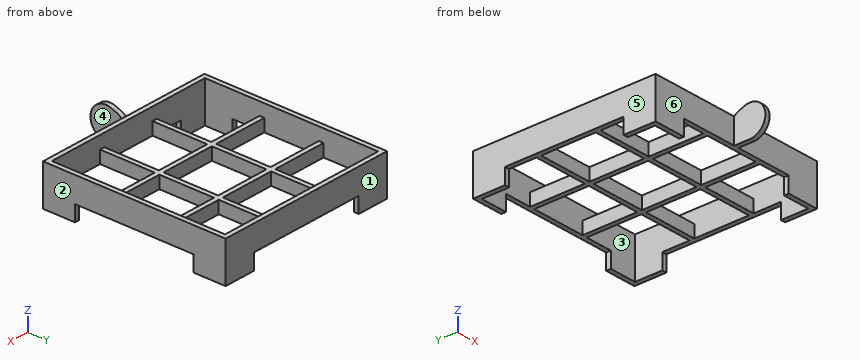
```python
from build123d import *

# Parameters (mm, degrees)
F0_W        = 58.5
F0_H        = 58.5
F0_W_2      = 17.5
F0_H_2      = 17.5
F1_DEPTH    = 4
F2_W        = 1.5
F2_H        = 10
F3_DEPTH    = 10
F4_R        = 4.99999
F6_DEPTH    = 1.5
F7_T1_DEPTH = 26.0435355486
F8_R        = 5
F9_W        = 58.5
F9_H        = 58.5
F9_W_2      = 55.5
F9_H_2      = 55.5
F10_DEPTH   = 4
F12_DEPTH   = 5


# Not quite as in the source:
# - a fillet or chamfer that OpenCascade refuses, or shapes differently, is made with other operations: its cross-section is extruded or revolved along the edge and cut away or added
# - a fillet or chamfer is up to 0.001 mm smaller than in the source, because OpenCascade refuses the exact size


with BuildPart() as f1:
    # F0 (on Top) → F1 (new body)
    with BuildSketch(Plane.XY):
        with Locations((-13.779699502, 7.1240415001)):
            Rectangle(F0_W, F0_H)
        with Locations((-32.779699502, -11.8759584999)):
            Rectangle(F0_W_2, F0_H_2, mode=Mode.SUBTRACT)
        with Locations((-13.779699502, -11.8759584999)):
            Rectangle(F0_W_2, F0_H_2, mode=Mode.SUBTRACT)
        with Locations((5.220300498, -11.8759584999)):
            Rectangle(F0_W_2, F0_H_2, mode=Mode.SUBTRACT)
        with Locations((-32.779699502, 7.1240415001)):
            Rectangle(F0_W_2, F0_H_2, mode=Mode.SUBTRACT)
        with Locations((-32.779699502, 26.1240415001)):
            Rectangle(F0_W_2, F0_H_2, mode=Mode.SUBTRACT)
        with Locations((-13.779699502, 7.1240415001)):
            Rectangle(F0_W_2, F0_H_2, mode=Mode.SUBTRACT)
        with Locations((5.220300498, 7.1240415001)):
            Rectangle(F0_W_2, F0_H_2, mode=Mode.SUBTRACT)
        with Locations((-13.779699502, 26.1240415001)):
            Rectangle(F0_W_2, F0_H_2, mode=Mode.SUBTRACT)
        with Locations((5.220300498, 26.1240415001)):
            Rectangle(F0_W_2, F0_H_2, mode=Mode.SUBTRACT)
    extrude(amount=F1_DEPTH)

    # F2 (on face) → F3 (join)
    with BuildSketch(Plane.XZ.offset(22.1259584999)):
        with Locations((-13.779699502, 5)):
            Rectangle(F2_W, F2_H)
    extrude(amount=F3_DEPTH)

    # F4 (radius 5 in the source; OpenCascade refuses exactly that, so slightly less here)
    f4_edges = [f1.edges().sort_by_distance(p)[0] for p in [
        (-13.7797, -32.125958, 10),
        (-13.7797, -32.125958, 0),
        (-13.7797, -22.125958, 10),
    ]]
    fillet(f4_edges, radius=F4_R)

    # F5 (on face) → F6 (join)
    with BuildSketch(Plane(origin=(-14.529699502, 0, 0), x_dir=(0, -1, 0), z_dir=(-1, 0, 0))):
        with BuildLine():
            Line((20.6259584999, 4), (22.1259584999, 4))
            Line((22.1259584999, 4), (22.1259584999, 5))
            ThreePointArc((22.1259584999, 5), (22.8099724149, 7.5243343902), (24.6748641453, 9.3579968409))
            Line((24.6748641453, 9.3579968409), (22.1259584999, 9.3579968409))
            Line((22.1259584999, 9.3579968409), (20.6259584999, 9.3579968409))
            Line((20.6259584999, 9.3579968409), (20.6259584999, 4))
        make_face()
    extrude(amount=-F6_DEPTH)

    # F7: fillet of radius 5 on 1 edges, made by hand

    # F7_s2 → F7_t1 (cut)
    with BuildSketch(Plane.YZ.offset(-26.8014672763)):
        with BuildLine():
            ThreePointArc((-20.6259584999, 4.4492897311), (-21.7687892868, 7.6308374145), (-24.6748567646, 9.3579968409))
            Line((-24.6748567646, 9.3579968409), (-24.6558347299, 9.4561709831))
            ThreePointArc((-24.6558347299, 9.4561709831), (-22.6504076323, 9.4579968409), (-20.6259584999, 9.4579968409))
            Line((-20.6259584999, 9.4579968409), (-20.5259584999, 9.3579968409))
            Line((-20.5259584999, 9.3579968409), (-20.5259584999, 4.4492897311))
            Line((-20.5259584999, 4.4492897311), (-20.6259584999, 4.4492897311))
        make_face()
    extrude(amount=F7_T1_DEPTH, mode=Mode.SUBTRACT)

    # F8
    f8_edges = [f1.edges().sort_by_distance(p)[0] for p in [
        (-13.7797, -24.674857, 9.357997),
    ]]
    fillet(f8_edges, radius=F8_R)

    # F9 (on face) → F10 (join)
    with BuildSketch(Plane.XY.offset(4)):
        with Locations((-13.779699502, 7.1240415001)):
            Rectangle(F9_W, F9_H)
        with Locations((-13.779699502, 7.1240415001)):
            Rectangle(F9_W_2, F9_H_2, mode=Mode.SUBTRACT)
    extrude(amount=F10_DEPTH)

    # F11 (on face) → F12 (join)
    with BuildSketch(Plane(origin=(0, 0, 0), x_dir=(1, 0, 0), z_dir=(0, 0, -1))):
        Polygon((-43.029699502, 11.8759584999), (-41.529699502, 11.8759584999), (-41.529699502, 20.6259584999), (-32.779699502, 20.6259584999), (-32.779699502, 22.1259584999), (-41.529699502, 22.1259584999), (-43.029699502, 22.1259584999), align=None)
        Polygon((5.220300498, 22.1259584999), (5.220300498, 20.6259584999), (13.970300498, 20.6259584999), (13.970300498, 11.8759584999), (15.470300498, 11.8759584999), (15.470300498, 22.1259584999), (13.970300498, 22.1259584999), align=None)
        Polygon((-43.029699502, -36.3740415001), (-32.779699502, -36.3740415001), (-32.779699502, -34.8740415001), (-41.529699502, -34.8740415001), (-41.529699502, -26.1240415001), (-43.029699502, -26.1240415001), (-43.029699502, -34.8740415001), align=None)
        Polygon((13.970300498, -34.8740415001), (5.220300498, -34.8740415001), (5.220300498, -36.3740415001), (15.470300498, -36.3740415001), (15.470300498, -34.8740415001), (15.470300498, -26.1240415001), (13.970300498, -26.1240415001), align=None)
    extrude(amount=F12_DEPTH)


solid = f1.part
```
Part model, mm, in its own coordinate system. Face numbers are marked on the shaded views. A direction names the side the tool comes from. Give positions to 0.01 mm unless a question says otherwise; leave off trailing zeros. Order: outer loops, then holes, each group sorted by start corner. A loop starts at its lowest first (then second) coordinate and runs counter-clockwise, first axis right, second up. Notation, with made-up numbers: M 71,41 L 88,41 A27 cw 88,75 Z; hole C 52.25,54 d3. An arc over 180 degrees is marked long. Use a Markdown table: item, result. Add a question column.
(1) 3-axis set-ups, long thin cutter, end or side, ignore diameter. For the marked faces 4, 5 and 6: which of +Z, -Z, +X, -X, +Y, -Y reach the whole face in a straight line?
(2) Saw through at B-B, the plane y = 7.5. Give the cut face in (x, z).
(3) Saw through at A-A, the plane x = 3. Give the cut face in (y, z).
(4) Saw through at D-D, the plane z = 2.5. Give the number of separate pieces and of enclosed holes in the cut face, and give its area (3 significant figures).
(5) Drop flat-ended pins along their axis: P1, Ø6, axis at x = -26.5, y = 27, coming from the -Z side; P2, Ø5, axis at x = -7.5, y = 15.5, coming from the +Z side; P3, Ø1.2, axis at x = -30, z = 3, coming from the -Y side. Give the stop position or say it passes through.
(6) Mould opens along X. For the marked faces 1, 2 and 3 say: +X half, -X half, draft (parallel to the pull), parting line (faces both ways), or undercut.
(7) Saw through at C-C, the plane z = 7. Give the cut face in (x, y).
(8) Probe line 1 along Y through (x, z) = (9, 1.75); line 2 along X through (y, z) = (-16, 0.5); line 3 along Y through (x, z) = (-28.5, 6.25). List the from-to ranges inside material, lowest first. Write a range as [from, to].
Answer key:
| question | item | result |
|---|---|---|
| 1 | face 4 | +Z, -Z, +X, -Y |
| 1 | face 5 | +Z, -Z, -X, +Y, -Y |
| 1 | face 6 | +Z, -Z, -X, -Y |
| 2 | outline | M -43.03,0 L -41.53,0 L -41.53,8 L -43.03,8 Z; M -24.03,0 L -22.53,0 L -22.53,4 L -24.03,4 Z; M -5.03,0 L -3.53,0 L -3.53,4 L -5.03,4 Z; M 13.97,0 L 15.47,0 L 15.47,8 L 13.97,8 Z |
| 3 | outline | M -22.13,0 L -20.63,0 L -20.63,8 L -22.13,8 Z; M -3.13,0 L -1.63,0 L -1.63,4 L -3.13,4 Z; M 15.87,0 L 17.37,0 L 17.37,4 L 15.87,4 Z; M 34.87,0 L 36.37,0 L 36.37,8 L 34.87,8 Z |
| 4 | separate pieces | 1 |
| 4 | enclosed holes | 9 |
| 4 | area | 680 mm^2 |
| 5 | P1 | z = 0 |
| 5 | P2 | z = 4 |
| 5 | P3 | y = -22.13 |
| 6 | face 1 | draft |
| 6 | face 2 | +X half |
| 6 | face 3 | undercut |
| 7 | outline | M -43.03,-22.13 L -14.53,-22.13 L -14.53,-31.71 L -13.03,-31.71 L -13.03,-22.13 L 15.47,-22.13 L 15.47,36.37 L -43.03,36.37 Z; hole M -41.53,-20.63 L 13.97,-20.63 L 13.97,34.87 L -41.53,34.87 Z |
| 8 | line 1 | [-22.13, -20.63], [-3.13, -1.63], [15.87, 17.37], [34.87, 36.37] |
| 8 | line 2 | [-43.03, -41.53], [-24.03, -22.53], [-5.03, -3.53], [13.97, 15.47] |
| 8 | line 3 | [-22.13, -20.63], [34.87, 36.37] |
